Model file for the job. Use its own axes, mm. Face numbers are marked on the shaded views. A direction names the side the tool comes from. Coordinates: 2 decimals unless noted, no trailing zeros. Write each loop counter-clockwise with the first axis right and the second up, starting at its lowest first coordinate (ties: lowest second). Pieces come first, ordered by that corner, then holes. Notation, with made-up numbers: M 69.5,54 L 89.5,54 A28 cw 89.5,93 Z; hole C -35,-29 d11. An arc over 180 degrees is marked long. Put each result on its own line as item: value. Start each with the question number.
Q1. Drill centre lines: line 1 along Z through (x, y) = (2.6, 2.5); line 2 along Y through (x, z) = (8, 1.7); line 3 along X through (y, z) = (-0.75, 0.6). Where is each one in solid material? Low to high.
Q2. Which spindle directions (+Z, -Z, +X, -X, +Y, -Y) get a long thin tool onto all of the face, cutting with end or side? Do the marked faces 5 and 6. Say none if no direction does.
Q3. Cut at B-B (x = 1.5). Write the cut outline in (y, z).
Q4. Cut at A-A (z = 3). Write the cut outline in (x, y), then the cut area to 3 significant figures.
Q5. Pull direction X, two halves, no side cores. Call the marked faces 1, 2, 3 and 4: pulls with the +X half, pulls with the -X half, needs draft (parallel to the pull), parting line crosses it, or undercut.
Q6. Drop flat-ended pins along their axis: pin 1 (5 mm diameter, centred on x = 10, y = 0, fed in from +Z); pin 2 (1 mm diameter, centred on x = 16, z = 1, fed in from +Y); pin 3 (3 mm diameter, centred on x = 2.6, z = 2.6, fed in from -Y). Give the stop position or say it passes through.
Autodesk Inventor part; units mm, degrees
ref_plane "YZ Plane" through (0, 0, 0) normal (1, 0, 0) x (0, 1, 0)
ref_plane "XZ Plane" through (0, 0, 0) normal (0, 1, 0) x (-1, 0, 0)
ref_plane "XY Plane" through (0, 0, 0) normal (0, 0, 1) x (1, 0, 0)
sketch "Sketch1" plane through (0, 0, 0) normal (0, 0, 1) x (1, 0, 0)
  line L0 (0, 0) -> (25, 0)
  line L1 (25, 0) -> (25, 6.2)
  line L2 (25, 6.2) -> (0, 6.2)
  line L3 (0, 6.2) -> (0, 0)
  point P0 (25, 3.1)
  dimension "d0" = 6.2
  dimension "d1" = 25
extrude "Extrusion1" add sketch "Sketch1" along normal blind 5.2
sketch "Sketch2" plane through (0, 0, 0) normal (0, -1, 0) x (1, 0, 0)
  circle A0 centre (2.6, 2.6) radius 1.6
  line L0 (0, 0) -> (0, 5.2)
  line L1 (0, 5.2) -> (25, 5.2)
  dimension "d4" = 3.2
  dimension "d5" = 2.6
  dimension "d6" = 2.6
extrude "Extrusion2" cut sketch "Sketch2" against normal blind 6.5
fillet "Fillet1" radius 2.6 2 edges at (0, 3.1, 5.2) (0, 3.1, 0)
sketch "Sketch4" plane through (2.6, 6.2, 0) normal (0, 1, 0) x (1, 0, 0)
  circle A0 centre (20.4, -2) radius 2
  line L0 (22.4, 0) -> (22.4, -5.2)
  line L1 (22.4, 0) -> (0, 0)
  point P0 (-2.6, 0)
  point P1 (27.4, -4)
  dimension "d13" = 4
  dimension "d14" = 2
  dimension "d15" = 2
extrude "Extrusion4" add sketch "Sketch4" along normal blind 5 and the other way blind 11.2 contours A0
sketch "Sketch5" plane through (2.6, 6.2, 5.2) normal (0, 1, 0) x (1, 0, 0)
  arc A0 (0, 5.2) -> (0, 0) centre (0, 2.6) ccw
  line L0 (0, 0) -> (22.4, 1.3139)
  line L1 (22.4, 3.2) -> (22.4, 0)
  circle A1 centre (20.4, 3.2) radius 2
  line L2 (22.4, 1.3139) -> (22.4, 0)
  line L3 (22.4, 0) -> (0, 0)
  circle A2 centre (20.4, 3.2) radius 2
  line L4 (22.4, 1.3139) -> (22.4, 3.2)
  point P0 (-2.6, 5.2)
  point P1 (20.5171, 1.2034)
extrude "Extrusion5" cut sketch "Sketch5" against normal blind 6.2 contours L0 L1 L3 | A1 L1 L0
fillet "Fillet2" radius 2 1 edges at (25, 3.1, 0)
properties part number "Latch"
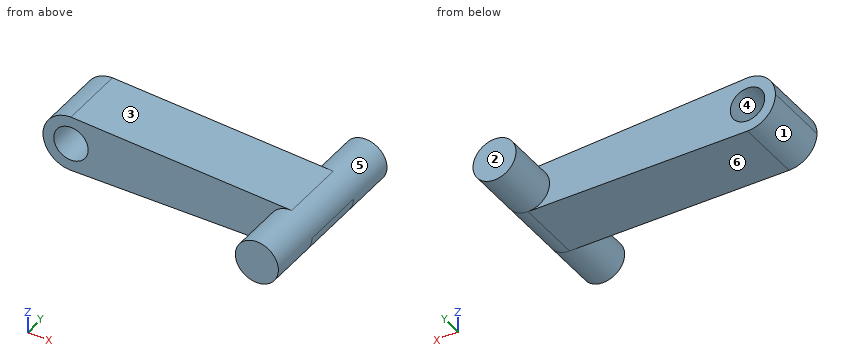
Computed values:
1. line 1: 0 to 1, 4.2 to 5.2
1. line 2: 0 to 6.2
1. line 3: 21.57 to 24.43
2. face 5: none
2. face 6: -Z, +X, -X, +Y, -Y
3. outline: M 0,0.24 L 6.2,0.24 L 6.2,1.44 L 0,1.44 Z; M 0,3.76 L 6.2,3.76 L 6.2,4.96 L 0,4.96 Z
4. outline: M 0.03,0 L 1.05,0 L 1.05,6.2 L 0.03,6.2 Z; M 4.15,0 L 21.27,0 L 21.27,-5 L 24.73,-5 L 24.73,11.2 L 21.27,11.2 L 21.27,6.2 L 4.15,6.2 Z
4. area: 169 mm2
5. face 1: pulls with the -X half
5. face 2: needs draft
5. face 3: pulls with the +X half
5. face 4: undercut
6. pin 1: z = 4.91
6. pin 2: y = 6.2
6. pin 3: through
